Read the model definition and answer for the solid it produces. Units are mm, in the model's axes. Face numbers are marked on the shaded views. A direction names the side the tool comes from. Round coordinates to 2 decimals unless told otherwise and drop trailing zeros. Order: outer loops, then holes, each group sorted by start corner. A loop starts at its lowest first (then second) coordinate and runs counter-clockwise, first axis right, second up. Notation, with made-up numbers: (84, -14) -> (100, -14) arc R32 cw to (100, 14) -> close; hole circle Ø2 at (-25.5, 37.5). An arc over 180 degrees is marked (long way). Answer as a JSON object with one key per item and string values. Group by question number.
Item 1: For the marked faces 1 and 2, determine the directions among +Z, -Z, +X, -X, +Y, -Y from which every point of the face is accessible in a straight line to the end or side of a thin tool.
Item 2: The mould has two halves that part along Z. Classify the marked faces 3, 4 and 5: pulls with the +Z half, pulls with the -Z half, needs draft (parallel to the pull), parting line crosses it, or undercut.
Item 3: Section C-C, the plane x = -76 is taken. Write down the section's boundary in (y, z).
Item 4: Section A-A, the plane y = 39.5 is taken. Write down the section's boundary in (x, z).
Item 5: Consider probe 1 along Z at (x, y) = (-254, 47.5); probe 2 along Y at (x, z) = (-297, -54.35); probe 3 along Y at (x, z) = (-14, 17). Determine where each line is inside the solid, lowest interval first. Write a range as from..to.
Item 6: Section B-B, the plane x = -320 is taken. Write down the section's boundary in (y, z).
Item 7: Section D-D, the plane y = 67 is taken. Write down the section's boundary in (x, z), plus the area to 3 significant figures.
Item 8: Given P1, Ø3, axis at x = -343, y = 29, coming from the -Z side; P2, Ø1, axis at x = -230, z = -20.5, coming from the +Y side, each flat-ended and moving along its own axis, determine where each tip first touches the part or whether it passes through.
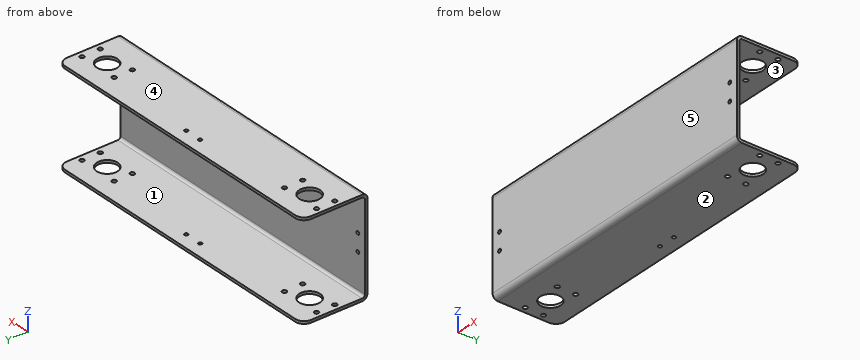
from build123d import *

# Parameters (mm, degrees)
SKETCH1_W                    = 350
SKETCH1_H                    = 100
BASE_FLANGE1_DEPTH           = 3
SM_EDGE_FLANGE_1_DEPTH       = 350
SM_EDGE_FLANGE_1_BEND_DEPTH  = 350
F_5_0_5_DIAMETER_HOLE1_D     = 5
SKETCH14_R                   = 12
CUT_EXTRUDE1_DEPTH           = 375.470292547
F_4_0_4_DIAMETER_HOLE1_D     = 4
F_4_0_4_DIAMETER_HOLE1_DEPTH = 3
F_4_0_4_DIAMETER_HOLE2_D     = 4
FILLET1_R                    = 10


# Sheet-metal steps are written as plain solids
with BuildPart() as part:
    # Sketch1 → Base-Flange1 (new body)
    with BuildSketch(Plane(origin=(0, 0, 0), x_dir=(1, 0, 0), z_dir=(0, 1, 0))):
        with Locations((-175, 0)):
            Rectangle(SKETCH1_W, SKETCH1_H)
    extrude(amount=-BASE_FLANGE1_DEPTH)

    # 邊線-凸緣1 section (across the edge) → 邊線-凸緣1 (add)
    with BuildSketch(Plane(origin=(-350, 0, 53), x_dir=(0, 0, -1), z_dir=(1, 0, 0))):
        with BuildLine():
            Line((-3, 3), (-3, 72))
            Line((-3, 72), (0, 72))
            Line((0, 72), (0, 3))
            ThreePointArc((0, 3), (0.878679656, 0.878679656), (3, 0))
            Line((3, 0), (3, -3))
            ThreePointArc((3, -3), (-1.242640687, -1.242640687), (-3, 3))
        make_face()
    extrude(amount=SM_EDGE_FLANGE_1_DEPTH)

    # 邊線-凸緣1 section 2 (across the edge) → 邊線-凸緣1 bend (add)
    with BuildSketch(Plane(origin=(0, 0, -53), x_dir=(0, 0, 1), z_dir=(-1, 0, 0))):
        with BuildLine():
            Line((-3, 3), (-3, 72))
            Line((-3, 72), (0, 72))
            Line((0, 72), (0, 3))
            ThreePointArc((0, 3), (0.878679656, 0.878679656), (3, 0))
            Line((3, 0), (3, -3))
            ThreePointArc((3, -3), (-1.242640687, -1.242640687), (-3, 3))
        make_face()
    extrude(amount=SM_EDGE_FLANGE_1_BEND_DEPTH)

    # Ø5.0 (5) Diameter Hole1 (through all)
    with Locations(Plane.XY.offset(56)):
        with Locations((-343, 50), (-343, 29), (-297, 50), (-297, 29)):
            f_5_0_5_diameter_hole1 = Hole(F_5_0_5_DIAMETER_HOLE1_D / 2)

    # Sketch14 → Cut-Extrude1 (cut, symmetric)
    with BuildSketch(Plane.XY.offset(56)):
        with Locations((-320, 39.5)):
            Circle(SKETCH14_R)
    cut_extrude1 = extrude(amount=CUT_EXTRUDE1_DEPTH, both=True, mode=Mode.SUBTRACT)

    # Mirror1: Ø5.0 (5) Diameter Hole1, Cut-Extrude1 across plane
    add(f_5_0_5_diameter_hole1.mirror(Plane(origin=(-175, 0, 0), x_dir=(0, 0, 1), z_dir=(1, 0, 0))), mode=Mode.SUBTRACT)
    add(cut_extrude1.mirror(Plane(origin=(-175, 0, 0), x_dir=(0, 0, 1), z_dir=(1, 0, 0))), mode=Mode.SUBTRACT)

    # Ø4.0 (4) Diameter Hole1
    with Locations(Plane.XY.offset(-53)):
        with Locations((-185, 57), (-165, 57)):
            f_4_0_4_diameter_hole1 = Hole(F_4_0_4_DIAMETER_HOLE1_D / 2, depth=F_4_0_4_DIAMETER_HOLE1_DEPTH)

    # Ø4.0 (4) Diameter Hole2 (through all)
    with Locations(Plane(origin=(0, 0, 0), x_dir=(1, 0, 0), z_dir=(0, 1, 0))):
        with Locations((-340, 10), (-340, -10)):
            f_4_0_4_diameter_hole2 = Hole(F_4_0_4_DIAMETER_HOLE2_D / 2)

    # Mirror2: Ø4.0 (4) Diameter Hole2 across plane
    add(f_4_0_4_diameter_hole2.mirror(Plane(origin=(-175, 0, 0), x_dir=(0, 0, 1), z_dir=(1, 0, 0))), mode=Mode.SUBTRACT)

    # Mirror3: Ø4.0 (4) Diameter Hole1 across plane
    add(f_4_0_4_diameter_hole1.mirror(Plane.XY), mode=Mode.SUBTRACT)

    # Fillet1
    fillet1_edges = [part.edges().sort_by_distance(p)[0] for p in [
        (-350, 72, 54.5),
        (0, 72, 54.5),
        (0, 72, -54.5),
        (-350, 72, -54.5),
    ]]
    fillet(fillet1_edges, radius=FILLET1_R)


solid = part.part
Values found:
{
 "1": {"face 1": "+X, -X, +Y", "face 2": "-Z, +X, -X, +Y, -Y"},
 "2": {"face 3": "undercut", "face 4": "pulls with the +Z half", "face 5": "needs draft"},
 "3": {"outline": "(-3, -50) arc R6 ccw to (3, -56) -> (72, -56) -> (72, -53) -> (3, -53) arc R3 cw to (0, -50) -> (0, 50) arc R3 cw to (3, 53) -> (72, 53) -> (72, 56) -> (3, 56) arc R6 ccw to (-3, 50) -> close"},
 "4": {"outline": "(-350, -56) -> (-332, -56) -> (-332, -53) -> (-350, -53) -> close; (-350, 53) -> (-332, 53) -> (-332, 56) -> (-350, 56) -> close; (-308, -56) -> (-42, -56) -> (-42, -53) -> (-308, -53) -> close; (-308, 53) -> (-42, 53) -> (-42, 56) -> (-308, 56) -> close; (-18, -56) -> (0, -56) -> (0, -53) -> (-18, -53) -> close; (-18, 53) -> (0, 53) -> (0, 56) -> (-18, 56) -> close"},
 "5": {"probe 1": "-56..-53, 53..56", "probe 2": "-1.13..26.5, 31.5..47.5, 52.5..72", "probe 3": "-3..0"},
 "6": {"outline": "(-3, -50) arc R6 ccw to (3, -56) -> (27.5, -56) -> (27.5, -53) -> (3, -53) arc R3 cw to (0, -50) -> (0, 50) arc R3 cw to (3, 53) -> (27.5, 53) -> (27.5, 56) -> (3, 56) arc R6 ccw to (-3, 50) -> close; (51.5, -56) -> (72, -56) -> (72, -53) -> (51.5, -53) -> close; (51.5, 53) -> (72, 53) -> (72, 56) -> (51.5, 56) -> close"},
 "7": {"outline": "(-348.66, -56) -> (-1.34, -56) -> (-1.34, -53) -> (-348.66, -53) -> close; (-348.66, 53) -> (-1.34, 53) -> (-1.34, 56) -> (-348.66, 56) -> close", "area": "2,080 mm2"},
 "8": {"P1": "through", "P2": "y = 0"}
}
